Design review of the part built by this model. Coordinates are the model's own, in mm. A direction names the side the tool comes from. Coordinates: 2 decimals unless noted, no trailing zeros. Loops run counter-clockwise (first coordinate to the right, second up) from the corner with the lowest first, then second, coordinate; pieces in that order, holes last. Notation, with made-up numbers: (41.5, 28.25) -> (64.5, 28.25) arc R22 cw to (64.5, 39.25) -> close; hole circle Ø3 at (-21.5, 3.25). An arc over 180 degrees is marked (long way). Use one line per item in the form item = value. Start each with the question number.
1. The part is to be moulded in two halves that separate along X. For faces 1 (the face through (152.4, -35, 2)), 2 (the face through (158.839, -35.381, -1.707)), 3 (the face through (93, 8, -6.35)), say which applies: released by +X, released by -X, zero draft, split by the parting line, or undercut.
2. Consider section D-D (y = 28). State the section outline as (x, z) points, then the cut area to 3 significant figures.
3. Machinability: for faces 4 (the face through (61, 11.748, 0)), 5 (the face through (77, -6.35, 5)), 6 (the face through (128.941, -14.554, 0.089)), which of the approach directions +Z, -Z, +X, -X, +Y, -Y give a long, thin tool a straight path to every point of the face, cutting with its end or side? Answer none if there is none.
4. For pin 1 (1.9 mm diameter, centred on x = 149, z = 1.5, fed in from -Y); pin 2 (2 mm diameter, centred on x = 10, y = -15, fed in from +Z) (3 decimals); pin 3 (3.5 mm diameter, centred on x = 85, z = 4.5, fed in from -Y); pin 4 (4 mm diameter, centred on x = 97, y = 0, fed in from -Z) (3 decimals), all flat-tipped, find the tip position at first contact; note any pin that passes through.
5. Consider section C-C (x = 0). State the section outline as (y, z) points (3 decimals).
6. Consider section A-A (z = 0). State how many separate pieces and enclosed holes the cut face has, then the cut area to 3 significant figures.
7. Consider section B-B (y = 0). State the section outline as (x, z) points (3 decimals), then the cut area to 3 significant figures.
8. Wall thickness on line 1 (X direction, y = 6, z = -10); line 2 (Y direction, x = 156.75, z = 0); line 3 (Z direction, x = 139.5, y = -22.5): over which ranges is each line inside the solid? List them lowest first. Write a range as from..to.
from build123d import *

# Parameters (mm, degrees)
BOSS_EXTRUDE2_DEPTH = 6.35
SKETCH2_8_R         = 15.875
SKETCH2_8_R_2       = 12.7
BOSS_EXTRUDE3_DEPTH = 12.7
SKETCH2_9_R         = 15.875
SKETCH2_9_R_2       = 12.7
BOSS_EXTRUDE4_DEPTH = 3.175
SKETCH3_R           = 3.175
BOSS_EXTRUDE6_DEPTH = 12.7


with BuildPart() as part:
    # Sketch2 → Boss-Extrude2 (new body, symmetric)
    with BuildSketch(Plane.XY):
        with BuildLine():
            Line((106.485681071, 11.7475), (14.793592152, 11.7475))
            ThreePointArc((14.793592152, 11.7475), (11.380569705, 12.214704826), (8.218662306, 13.581944444))
            ThreePointArc((8.218662306, 13.581944444), (13.829079671, 7.79565138), (15.875, 0))
            ThreePointArc((15.875, 0), (14.696781618, -6.001686018), (11.33701763, -11.1125))
            ThreePointArc((11.33701763, -11.1125), (15.487942885, -8.293678539), (20.406631735, -7.3025))
            Line((20.406631735, -7.3025), (106.48193654, -7.3025))
            ThreePointArc((106.48193654, -7.3025), (129.228859651, -14.730836392), (146.05, -31.75))
            Line((146.05, -31.75), (165.1, -31.75))
            ThreePointArc((165.1, -31.75), (133.35, 0), (165.1, 31.75))
            Line((165.1, 31.75), (146.05, 31.75))
            ThreePointArc((146.05, 31.75), (128.565457442, 17.204135674), (106.485681071, 11.7475))
        make_face()
        with BuildLine():
            ThreePointArc((38.712408675, -6.35), (32.362408675, 0), (38.712408675, 6.35))
            Line((38.712408675, 6.35), (114.912408675, 6.35))
            ThreePointArc((114.912408675, 6.35), (121.262408675, 0), (114.912408675, -6.35))
            Line((114.912408675, -6.35), (38.712408675, -6.35))
        make_face(mode=Mode.SUBTRACT)
    extrude(amount=BOSS_EXTRUDE2_DEPTH, both=True)

    # Sketch2_8 → Boss-Extrude3 (add, symmetric)
    with BuildSketch(Plane.XY):
        Circle(SKETCH2_8_R)
        Circle(SKETCH2_8_R_2, mode=Mode.SUBTRACT)
        with BuildLine():
            Line((165.1, -25.4), (165.1, -31.75))
            ThreePointArc((165.1, -31.75), (133.35, 0), (165.1, 31.75))
            Line((165.1, 31.75), (165.1, 25.4))
            ThreePointArc((165.1, 25.4), (139.7, 0), (165.1, -25.4))
        make_face()
    extrude(amount=BOSS_EXTRUDE3_DEPTH, both=True)

    # Sketch2_9 → Boss-Extrude4 (add, symmetric)
    with BuildSketch(Plane.XY):
        Circle(SKETCH2_9_R)
        Circle(SKETCH2_9_R_2, mode=Mode.SUBTRACT)
        with BuildLine():
            Line((165.1, -25.4), (165.1, -31.75))
            ThreePointArc((165.1, -31.75), (133.35, 0), (165.1, 31.75))
            Line((165.1, 31.75), (165.1, 25.4))
            ThreePointArc((165.1, 25.4), (139.7, 0), (165.1, -25.4))
        make_face()
        with BuildLine():
            Line((38.712408675, 6.35), (114.912408675, 6.35))
            ThreePointArc((114.912408675, 6.35), (121.262408675, 0), (114.912408675, -6.35))
            Line((114.912408675, -6.35), (38.712408675, -6.35))
            ThreePointArc((38.712408675, -6.35), (32.362408675, 0), (38.712408675, 6.35))
        make_face()
    extrude(amount=BOSS_EXTRUDE4_DEPTH, both=True)

    # Sketch3 → Boss-Extrude6 (add)
    with BuildSketch(Plane(origin=(165.1, 0, 0), x_dir=(0, 0, -1), z_dir=(1, 0, 0))):
        with BuildLine():
            Line((6.35, 31.75), (6.35, 38.085125464))
            ThreePointArc((6.35, 38.085125464), (0, 44.435125464), (-6.35, 38.085125464))
            Line((-6.35, 38.085125464), (-6.35, 31.75))
            Line((-6.35, 31.75), (6.35, 31.75))
        make_face()
        with Locations((0, 38.085125464)):
            Circle(SKETCH3_R, mode=Mode.SUBTRACT)
        with BuildLine():
            Line((-6.35, -31.75), (-6.35, -38.058434683))
            ThreePointArc((-6.35, -38.058434683), (0, -44.408434683), (6.35, -38.058434683))
            Line((6.35, -38.058434683), (6.35, -31.75))
            Line((6.35, -31.75), (-6.35, -31.75))
        make_face()
        with Locations((0, -38.058434683)):
            Circle(SKETCH3_R, mode=Mode.SUBTRACT)
    extrude(amount=-BOSS_EXTRUDE6_DEPTH)


solid = part.part
Geometry check:
q1.face_1 = released by -X
q1.face_2 = zero draft
q1.face_3 = undercut
q2.outline = (142.9, -6.35) -> (150.13, -6.35) -> (150.13, -12.7) -> (165.1, -12.7) -> (165.1, 12.7) -> (150.13, 12.7) -> (150.13, 6.35) -> (142.9, 6.35) -> close
q2.area = 472 mm²
q3.face_4 = +Z, -Z, +Y
q3.face_5 = +Z
q3.face_6 = +Z, -Z, -Y
q4.pin_1 = -31.75
q4.pin_2 = through
q4.pin_3 = -7.3
q4.pin_4 = -3.175
q5.outline = (-15.875, -12.7) -> (-12.7, -12.7) -> (-12.7, 12.7) -> (-15.875, 12.7) -> close; (12.7, -12.7) -> (15.875, -12.7) -> (15.875, 12.7) -> (12.7, 12.7) -> close
q6.separate_pieces = 3
q6.enclosed_holes = 1
q6.area = 3,700 mm²
q7.outline = (-15.875, -12.7) -> (-12.7, -12.7) -> (-12.7, 12.7) -> (-15.875, 12.7) -> close; (12.7, -12.7) -> (15.875, -12.7) -> (15.875, -6.35) -> (32.362, -6.35) -> (32.362, -3.175) -> (121.262, -3.175) -> (121.262, -6.35) -> (133.35, -6.35) -> (133.35, -12.7) -> (139.7, -12.7) -> (139.7, 12.7) -> (133.35, 12.7) -> (133.35, 6.35) -> (121.262, 6.35) -> (121.262, 3.175) -> (32.362, 3.175) -> (32.362, 6.35) -> (15.875, 6.35) -> (15.875, 12.7) -> (12.7, 12.7) -> close
q7.area = 1,250 mm²
q8.line_1 = -14.7..-11.19, 11.19..14.7, 133.92..140.42
q8.line_2 = -44.41..-41.23, -34.88..-23.99, 23.99..34.91, 41.26..44.44
q8.line_3 = -6.35..6.35
